```python
from build123d import *

# Parameters (mm, degrees)
SKETCH1_W           = 38
SKETCH1_H           = 13
BOSS_EXTRUDE1_DEPTH = 12
SKETCH2_R           = 12
CUT_EXTRUDE1_DEPTH  = 13
HOLE1_D             = 2.35


with BuildPart() as part:
    # Sketch1 → Boss-Extrude1 (new body)
    with BuildSketch(Plane(origin=(0, 0, 0), x_dir=(1, 0, 0), z_dir=(0, 1, 0))):
        with Locations((19, 6.5)):
            Rectangle(SKETCH1_W, SKETCH1_H)
    extrude(amount=BOSS_EXTRUDE1_DEPTH)

    # Sketch2 → Cut-Extrude1 (cut)
    with BuildSketch(Plane.XY):
        with Locations((19, 16)):
            Circle(SKETCH2_R)
    extrude(amount=-CUT_EXTRUDE1_DEPTH, mode=Mode.SUBTRACT)

    # Hole1 (through all)
    with Locations(Plane(origin=(0, 0, 0), x_dir=(-1, 0, 0), z_dir=(0, -1, 0))):
        with Locations((-34, 6.5), (-4, 6.5)):
            Hole(HOLE1_D / 2)


solid = part.part
```
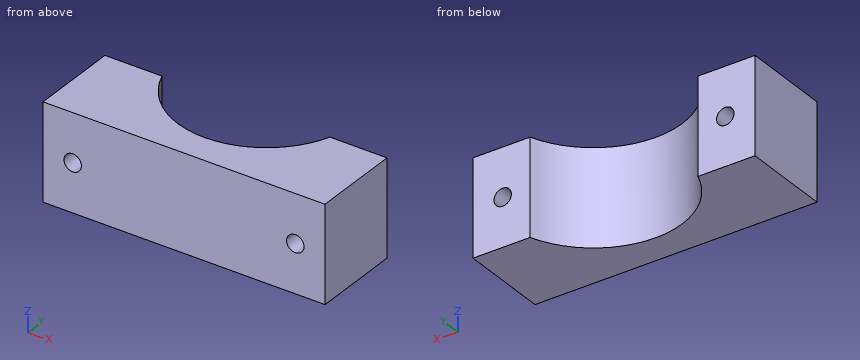
Can you work these out from the model? Positions are in its coordinate system, mm. Give positions to 0.01 mm unless a question says otherwise; leave off trailing zeros. Write each loop counter-clockwise with the first axis right and the second up, starting at its lowest first coordinate (ties: lowest second). Pieces come first, ordered by that corner, then holes. Notation, with made-up numbers: (71, -21.5) -> (77, -21.5) arc R27 ccw to (77, -3.5) -> close; hole circle Ø3 at (-29.5, 51.25). An arc over 180 degrees is marked (long way). One line per item, written item: value.
Q1. Imagine slicing it at A-A on y = 8.5. Give the number of separate pieces and of enclosed holes in the cut face, and give its area (3 significant figures).
Results found:
separate pieces: 2
enclosed holes: 2
area: 242 mm^2
Q2. Imagine slicing it at D-D on y = 1.75. Please give me the cut outline in (x, z) (3 decimals).
Results found:
outline: (0, -13) -> (38, -13) -> (38, 0) -> (0, 0) -> close; hole circle Ø2.35 at (4, -6.5); hole circle Ø2.35 at (34, -6.5)
Q3. For P1, Ø4, axis at y = 5.5, z = -6, coming from the -X side; P2, Ø1.5, axis at x = 16, z = -3.5, coming from the +Y side; P3, Ø1, axis at x = 27.5, z = -10.5, coming from the +Y side, each with a flat end and sliding along its axis, tell me the tip position at first contact or that it passes through.
Results found:
P1: stops at x = 0
P2: stops at y = 4.6
P3: stops at y = 8.06
Q4. Please list where these lines run through material, in increasing order: line 1 (X direction, y = 3.75, z = -6.5) (3 decimals); line 2 (X direction, y = 6.5, z = -6.5) (3 decimals); line 3 (X direction, y = 5, z = -6.5) (3 decimals). Write a range as [from, to].
Results found:
line 1: x = [0, 2.825], [5.175, 32.825], [35.175, 38]
line 2: x = [0, 2.825], [5.175, 11.669], [26.331, 32.825], [35.175, 38]
line 3: x = [0, 2.825], [5.175, 14.204], [23.796, 32.825], [35.175, 38]
Q5. Imagine slicing it at B-B on z = -6.5. Please give me the cut outline in (x, y) (3 decimals).
Results found:
outline: (0, 0) -> (2.825, 0) -> (2.825, 12) -> (0, 12) -> close; (5.175, 0) -> (32.825, 0) -> (32.825, 12) -> (30.314, 12) arc R12 cw to (7.686, 12) -> (5.175, 12) -> close; (35.175, 0) -> (38, 0) -> (38, 12) -> (35.175, 12) -> close
Q6. Imagine slicing it at C-C on x = 4. Please give me the cut outline in (y, z) (3 decimals), and give its area (3 significant figures).
Results found:
outline: (0, -13) -> (12, -13) -> (12, -7.675) -> (0, -7.675) -> close; (0, -5.325) -> (12, -5.325) -> (12, 0) -> (0, 0) -> close
area: 128 mm^2
